Answer from the drawing. Dimensions are ordinates in mm from the lowest x, y and z of the part. A direction names the side the tool comes from. Round coordinates to 2 decimals unless told otherwise and drop trailing zeros. Write each loop counter-clockwise with the first axis right and the second up, starting at its lowest first coordinate (ties: lowest second). Pieces come first, ordered by that corner, then holes. Notation, with made-up numbers: (25.5, -16.75) -> (80.5, -16.75) arc R13 ccw to (80.5, -11.75) -> close; hole circle Ø1 at (40.5, 25). An arc over 180 degrees is marked (long way). Return JSON: item names as keys, results as strings. Group by question number.
(1) The mould has two halves that part along Y. Classify the marked faces 1, 2, 3 and 4: released by +Y, released by -Y, zero draft, split by the parting line, or undercut.
(2) A cutting plane is placed at A-A on y = 9. Give the vertices of the cut face in (x, z).
(3) A cutting plane is placed at D-D on y = 12.75. Give the vertices of the cut face in (x, z), then the cut area to 3 significant figures.
(4) A cutting plane is placed at B-B on x = 14.5. Give the vertices of the cut face in (y, z).
(5) For the marked faces 5, 6 and 7, determine the directions among +Z, -Z, +X, -X, +Y, -Y from which every point of the face is accessible in a straight line to the end or side of a thin tool.
(6) Straight lines are drawn through the part: line 1 (Y direction, x = 7, z = 2.1); line 2 (X direction, y = 10.5, z = 2.25); line 3 (X direction, y = 11.25, z = 2.2). For each, find the intervals that lie inside material, in ascending order.
(7) A cutting plane is placed at C-C on z = 0.9. Give the vertices of the cut face in (x, y), then the cut area to 3 significant figures.
(8) Given pin 1 (0.8 mm diameter, centred on y = 2, z = 0.5, fed in from +X); pin 2 (0.8 mm diameter, centred on y = 2.5, z = 1, fed in from -X); pin 3 (0.8 mm diameter, centred on x = 1.5, z = 1, fed in from -Y), each flat-ended and moving along its own axis, determine where each tip first touches the part or whether it passes through.
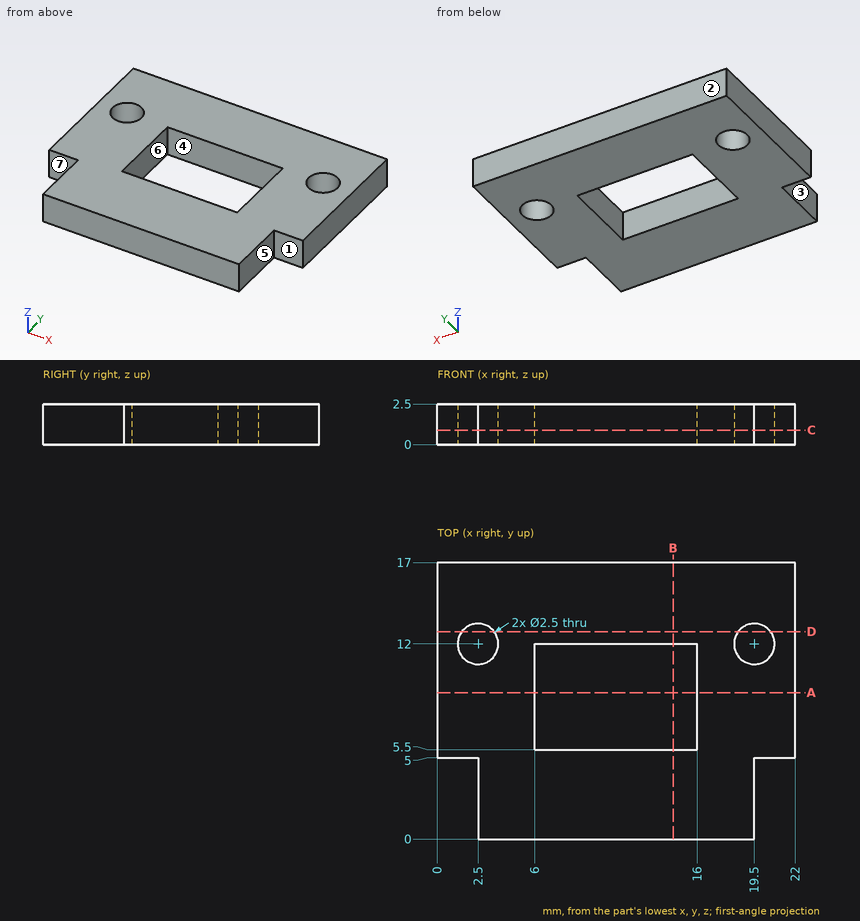
Checks:
{
 "1": {"face 1": "released by -Y", "face 2": "released by +Y", "face 3": "zero draft", "face 4": "undercut"},
 "2": {"outline": "(0, 0) -> (6, 0) -> (6, 2.5) -> (0, 2.5) -> close; (16, 0) -> (22, 0) -> (22, 2.5) -> (16, 2.5) -> close"},
 "3": {"outline": "(0, 0) -> (1.5, 0) -> (1.5, 2.5) -> (0, 2.5) -> close; (3.5, 0) -> (18.5, 0) -> (18.5, 2.5) -> (3.5, 2.5) -> close; (20.5, 0) -> (22, 0) -> (22, 2.5) -> (20.5, 2.5) -> close", "area": "45.0 mm^2"},
 "4": {"outline": "(0, 0) -> (5.5, 0) -> (5.5, 2.5) -> (0, 2.5) -> close; (12, 0) -> (17, 0) -> (17, 2.5) -> (12, 2.5) -> close"},
 "5": {"face 5": "+Z, -Z, +X, -Y", "face 6": "+Z, -Z", "face 7": "+Z, -Z, -X, -Y"},
 "6": {"line 1": "y = 0 to 5.5, 12 to 17", "line 2": "x = 0 to 6, 16 to 22", "line 3": "x = 0 to 1.5, 3.5 to 6, 16 to 18.5, 20.5 to 22"},
 "7": {"outline": "(0, 5) -> (2.5, 5) -> (2.5, 0) -> (19.5, 0) -> (19.5, 5) -> (22, 5) -> (22, 17) -> (0, 17) -> close; hole circle Ø2.5 at (2.5, 12); hole (6, 5.5) -> (16, 5.5) -> (16, 12) -> (6, 12) -> close; hole circle Ø2.5 at (19.5, 12)", "area": "274 mm^2"},
 "8": {"pin 1": "stops at x = 19.5", "pin 2": "stops at x = 2.5", "pin 3": "stops at y = 5"}
}
